Check sheet for the modelled part. Datum: model origin and axes. Units: mm. A direction names the side the tool comes from. Round coordinates to 2 decimals unless told otherwise and drop trailing zeros. Write each loop counter-clockwise with the first axis right and the second up, starting at its lowest first coordinate (ties: lowest second). Pieces come first, ordered by that corner, then holes. Notation, with made-up numbers: (7, 45) - (49, 45) arc R18 ccw to (49, 73) - close; hole circle Ø6 at (0.5, 10). An arc over 180 degrees is marked (long way). Use one line per item in the form item = value. Start each with the question number.
1) Scan lines: probe 1 along X at (y, z) = (49.5, -10); probe 2 along Y at (x, z) = (-46, -34.5); probe 3 along Z at (x, y) = (29, 37.5). Record each from-to range of solid material in increasing order.
2) Section check D-D (x = 71). Record the boundary of the cut face in (y, z).
3) Set-up check for faces 1 (the face through (2, 76, 10.976)), 2 (the face through (54.066, 36, -45)): record each of +Z, -Z, +X, -X, +Y, -Y from which the full face is reachable in a straight line by a thin tool's end or side.
4) Draft check along X on faces 3 (the face through (2, 101.6, -39)), 4 (the face through (104.866, 61, -52)), 5 (the face through (-47.534, 36, -45)), 6 (the face through (3, 50.8, -27)). Enter one of: +X half, -X half, draft (parallel to the pull), parting line (faces both ways), or undercut.
5) Section check C-C (z = -51). Record the boundary of the cut face in (x, y), then the cut area to 3 significant figures.
6) Section check A-A (x = -36.5). Record the boundary of the cut face in (y, z), then the cut area to 3 significant figures.
7) Section check B-B (y = 41.5). Record the boundary of the cut face in (x, z), then the cut area to 3 significant figures.
8) Gauge pin test, flat ends, axial feed: P1, Ø1, axis at x = -33.5, y = 40.5, coming from the +Z side; P2, Ø5, axis at x = 74, y = 41.5, coming from the +Z side. Record the tip position at first contact, or that the pin passes through.
from build123d import *

# Parameters (mm, degrees)
F0_W     = 203.2
F0_H     = 101.6
F1_DEPTH = 101.6
F2_SIZE2 = 76.2
F2_SIZE  = 50.8
F3_W     = 101.6
F3_H     = 76.2
F4_DEPTH = 50.8


with BuildPart() as f1:
    # F0 (on Front) → F1 (new body)
    with BuildSketch(Plane.XZ):
        with Locations((3.265716, -39.823574)):
            Rectangle(F0_W, F0_H)
    extrude(amount=-F1_DEPTH)

    # F2
    f2_edges = [f1.edges().sort_by_distance(p)[0] for p in [
        (3.265716, 0, 10.976426),
    ]]
    chamfer(f2_edges, length=F2_SIZE, length2=F2_SIZE2)

    # F3 (on Front) → F4 (cut)
    with BuildSketch(Plane.XZ):
        with Locations((3.265716, -27.022086)):
            Rectangle(F3_W, F3_H)
    extrude(amount=-F4_DEPTH, mode=Mode.SUBTRACT)


solid = f1.part
Results are:
q1.probe_1 = -98.33 to -47.53, 54.07 to 104.87
q1.probe_2 = 50.8 to 101.6
q1.probe_3 = -90.62 to -65.12
q2.outline = (0, -90.62) - (101.6, -90.62) - (101.6, 10.98) - (50.8, 10.98) - (0, -65.22) - close
q3.face_1 = +Z, +X, -X, +Y, -Y
q3.face_2 = +Z, -Y
q4.face_3 = draft
q4.face_4 = +X half
q4.face_5 = undercut
q4.face_6 = undercut
q5.outline = (-98.33, 9.48) - (-47.53, 9.48) - (-47.53, 50.8) - (54.07, 50.8) - (54.07, 9.48) - (104.87, 9.48) - (104.87, 101.6) - (-98.33, 101.6) - close
q5.area = 14,500 mm²
q6.outline = (0, -90.62) - (101.6, -90.62) - (101.6, 10.98) - (50.8, 10.98) - (50.8, -65.12) - (0.07, -65.12) - (0, -65.22) - close
q6.area = 6,460 mm²
q7.outline = (-98.33, -90.62) - (104.87, -90.62) - (104.87, -2.97) - (54.07, -2.97) - (54.07, -65.12) - (-47.53, -65.12) - (-47.53, -2.97) - (-98.33, -2.97) - close
q7.area = 11,500 mm²
q8.P1 = -65.12
q8.P2 = 0.78
